Part model, mm, in its own coordinate system. Face numbers are marked on the shaded views. A direction names the side the tool comes from. Coordinates: 2 decimals unless noted, no trailing zeros. Loops run counter-clockwise (first coordinate to the right, second up) from the corner with the lowest first, then second, coordinate; pieces in that order, holes last. Notation, with made-up numbers: (-19, -6.75) - (9, -6.75) arc R34 ccw to (9, 30.25) - close; hole circle Ø9 at (5, -17). An arc over 180 degrees is marked (long way). Use a Markdown table: item, result. Add a question column.
1) Band-saw the part on D-D (x = -3). Give the cut face in (y, z) (3 decimals), plus the area to 3 significant figures.
2) Drop flat-ended pins along their axis: P1, Ø8, axis at x = 0.5, y = 0.5, coming from the -Z side; P2, Ø5.5, axis at y = 10, z = 6.5, coming from the +X side; P3, Ø5.5, axis at x = 0, y = 0, coming from the +Z side; P4, Ø5, axis at y = 8.475, z = 7.5, coming from the +X side. Give the stop position or say it passes through.
3) Band-saw the part on A-A (z = 7.5). Give the cut face in (x, y) (3 decimals).
4) Band-saw the part on C-C (y = 7). Give the cut face in (x, z).
5) Probe probe 1 along Y at (x, z) = (-3.5, 4.5); probe 2 along Y at (x, z) = (0, 2.1); probe 3 along X at (y, z) = (10.5, 8.5). List the from-to ranges inside material, lowest first. Write a range as [from, to].
6) Tool access for the marked faces 1, 2 and 3: list every direction of +Z, -Z, +X, -X, +Y, -Y with a clear straight run to the whole face (end or side of a thin tool).
7) Pull direction Y, two halves, no side cores. Call the marked faces 4, 5 and 6: +Y half, -Y half, draft (parallel to the pull), parting line (faces both ways), or undercut.
8) Band-saw the part on B-B (x = 1.25). Give the cut face in (y, z) (3 decimals), plus the area to 3 significant figures.
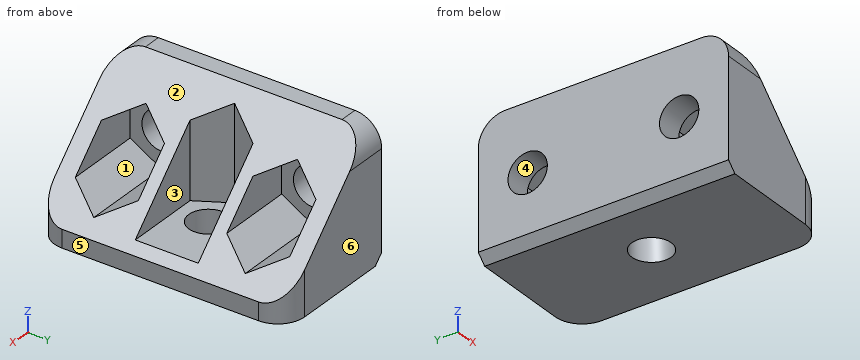
from build123d import *

# Parameters (mm, degrees)
SKETCH_W        = 15
SKETCH_H        = 28
PAD_DEPTH       = 15
SKETCH001_R     = 2.2
POCKET_DEPTH    = 15.001
POCKET001_DEPTH = 12
SKETCH003_R     = 2.2
POCKET002_DEPTH = 15.001
POCKET003_DEPTH = 12
POCKET004_DEPTH = 28.001
FILLET_R        = 3
CHAMFER_SIZE    = 1


with BuildPart() as part:
    # Sketch → Pad (new body)
    with BuildSketch(Plane.XY):
        Rectangle(SKETCH_W, SKETCH_H)
    extrude(amount=PAD_DEPTH)

    # Sketch001 → Pocket (cut, through all)
    with BuildSketch(Plane.YZ.offset(7.5)):
        with Locations((-8.475, 7.5)):
            Circle(SKETCH001_R)
        with Locations((8.475, 7.5)):
            Circle(SKETCH001_R)
    extrude(amount=-POCKET_DEPTH, mode=Mode.SUBTRACT)

    # Sketch002 → Pocket001 (cut)
    with BuildSketch(Plane.YZ.offset(7.5)):
        Polygon((-8.475, 3.429681), (-4.95, 5.46484), (-4.95, 9.53516), (-8.475, 11.570319), (-12, 9.53516), (-12, 5.46484), align=None)
        Polygon((8.475, 3.429681), (12, 5.46484), (12, 9.53516), (8.475, 11.570319), (4.95, 9.53516), (4.95, 5.46484), align=None)
    extrude(amount=-POCKET001_DEPTH, mode=Mode.SUBTRACT)

    # Sketch003 → Pocket002 (cut, through all)
    with BuildSketch(Plane.XY.offset(15)):
        Circle(SKETCH003_R)
    extrude(amount=-POCKET002_DEPTH, mode=Mode.SUBTRACT)

    # Sketch004 → Pocket003 (cut)
    with BuildSketch(Plane.XY.offset(15)):
        Polygon((2.03516, 3.525), (-2.03516, 3.525), (-4.070319, 0), (-2.03516, -3.525), (2.03516, -3.525), (7.53516, -3.525), (7.53516, 3.525), align=None)
    extrude(amount=-POCKET003_DEPTH, mode=Mode.SUBTRACT)

    # Sketch005 → Pocket004 (cut, through all)
    with BuildSketch(Plane.XZ.offset(14)):
        Polygon((7.5, 15), (7.5, 2), (-5.5, 15), align=None)
    extrude(amount=-POCKET004_DEPTH, mode=Mode.SUBTRACT)

    # Fillet
    fillet_edges = [part.edges().sort_by_distance(p)[0] for p in [
        (7.5, 14, 1),
        (7.5, -14, 1),
        (-6.5, -14, 15),
        (-6.5, 14, 15),
    ]]
    fillet(fillet_edges, radius=FILLET_R)

    # Chamfer
    chamfer_edges = [part.edges().sort_by_distance(p)[0] for p in [
        (-7.5, 0, 0),
    ]]
    chamfer(chamfer_edges, length=CHAMFER_SIZE)


solid = part.part
Answer block:
| question | item | result |
|---|---|---|
| 1 | outline | (-14, 0) - (14, 0) - (14, 12) arc R3 ccw to (13.958, 12.5) - (1.854, 12.5) - (1.854, 3) - (-1.854, 3) - (-1.854, 12.5) - (-13.958, 12.5) arc R3 ccw to (-14, 12) - close; hole (-12, 5.465) - (-8.475, 3.43) - (-4.95, 5.465) - (-4.95, 9.535) - (-8.475, 11.57) - (-12, 9.535) - close; hole (4.95, 5.465) - (8.475, 3.43) - (12, 5.465) - (12, 9.535) - (8.475, 11.57) - (4.95, 9.535) - close |
| 1 | area | 229 mm2 |
| 2 | P1 | z = 0 |
| 2 | P2 | x = 5.75 |
| 2 | P3 | z = 3 |
| 2 | P4 | x = -4.5 |
| 3 | outline | (-7.5, -14) - (2, -14) - (2, -12) - (-4.5, -12) - (-4.5, -10.675) - (-7.5, -10.675) - close; (-7.5, -6.275) - (-4.5, -6.275) - (-4.5, -4.95) - (2, -4.95) - (2, -3.525) - (-2.035, -3.525) - (-4.07, 0) - (-2.035, 3.525) - (2, 3.525) - (2, 4.95) - (-4.5, 4.95) - (-4.5, 6.275) - (-7.5, 6.275) - close; (-7.5, 10.675) - (-4.5, 10.675) - (-4.5, 12) - (2, 12) - (2, 14) - (-7.5, 14) - close |
| 4 | outline | (-7.5, 1) - (-6.5, 0) - (7.5, 0) - (7.5, 2) - (5.22, 4.28) - (-4.5, 4.28) - (-4.5, 5.87) - (-7.5, 5.87) - close; (-7.5, 9.13) - (-4.5, 9.13) - (-4.5, 10.72) - (-1.22, 10.72) - (-5.5, 15) - (-7.5, 15) - close |
| 5 | probe 1 | [-14, -10.33], [-6.62, -0.99], [0.99, 6.62], [10.33, 14] |
| 5 | probe 2 | [-14, -2.2], [2.2, 14] |
| 5 | probe 3 | [-7.5, -4.5] |
| 6 | face 1 | +X |
| 6 | face 2 | +Z, +X, +Y, -Y |
| 6 | face 3 | +Z, +X |
| 7 | face 4 | undercut |
| 7 | face 5 | draft |
| 7 | face 6 | +Y half |
| 8 | outline | (-14, 0) - (-1.81, 0) - (-1.81, 3) - (-3.525, 3) - (-3.525, 8.25) - (-4.95, 8.25) - (-4.95, 5.465) - (-8.475, 3.43) - (-12, 5.465) - (-12, 8.25) - (-14, 8.25) - close; (1.81, 0) - (14, 0) - (14, 8.25) - (12, 8.25) - (12, 5.465) - (8.475, 3.43) - (4.95, 5.465) - (4.95, 8.25) - (3.525, 8.25) - (3.525, 3) - (1.81, 3) - close |
| 8 | area | 130 mm2 |
